Job drawing, mm, ordinate dimensions from the low corner. One solid piece. A direction names the side the tool comes from. Give positions to 0.01 mm unless a question says otherwise; leave off trailing zeros. Write each loop counter-clockwise with the first axis right and the second up, starting at its lowest first coordinate (ties: lowest second). Pieces come first, ordered by that corner, then holes. Notation, with made-up numbers: (79.5, 16.5) - (107.5, 16.5) arc R7 cw to (107.5, 24.5) - close; hole circle Ø5 at (-28.75, 55). An arc over 180 degrees is marked (long way). Use a Markdown table: item, result. Add a question column.
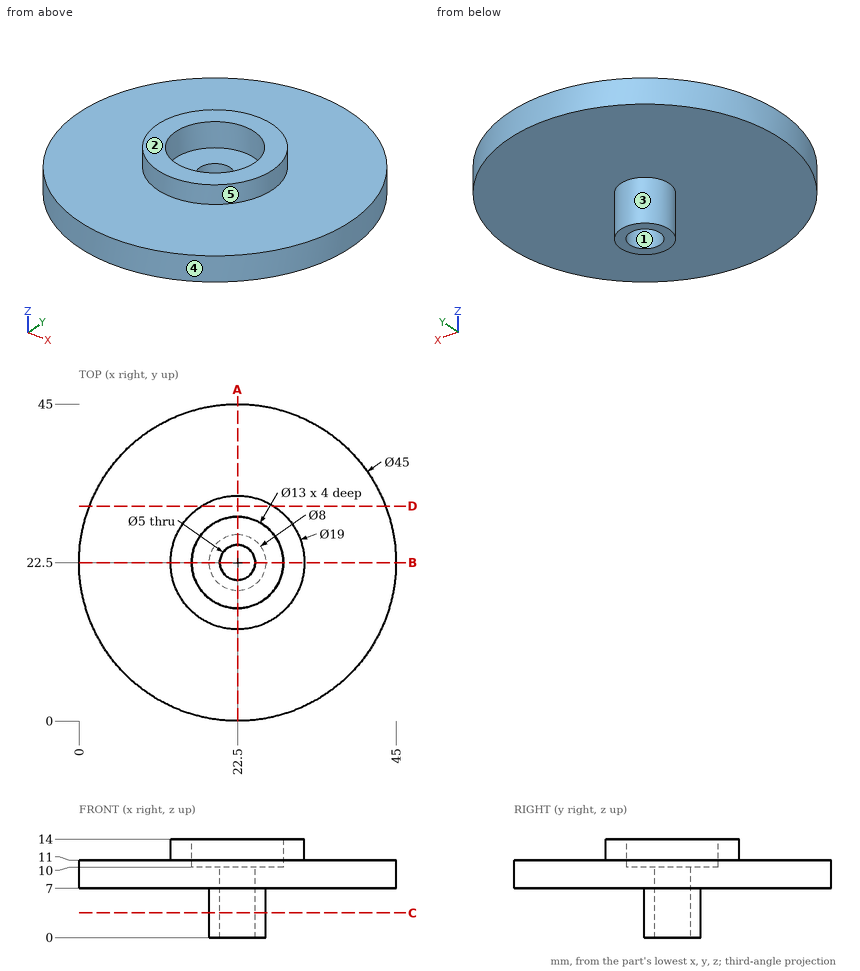
(1) Band-saw the part on C-C (z = 3.5). Write the cut outline in (x, y), then the cut area to 3 significant figures.
(2) Flat gauge pins, fed straight in: pin 1 (1 mm diameter, centred on y = 35.5, z = 9, fed in from -X); pin 2 (6 mm diameter, centred on y = 26, z = 7, fed in from -X); pin 3 (6 mm diameter, centred on y = 7.5, z = 12, fed in from +X). Where does each tip first touch, or does it go through?
(3) Band-saw the part on D-D (y = 30.5). Write the cut outline in (x, z).
(4) Probe probe 1 along X at (y, z) = (22.5, 12.9); probe 2 along Z at (x, y) = (30.5, 30); probe 3 along X at (y, z) = (22.5, 4.5). List the from-to ranges inside material, lowest first. Write a range as [from, to].
(5) Two-plate mould, pull along X, no slides. Class the marked faces 1, 2 and 3: +X half, -X half, draft (parallel to the pull), parting line (faces both ways), or undercut.
(6) Which spindle directions (+Z, -Z, +X, -X, +Y, -Y) get a long thin tool onto all of the face, cutting with end or side? Do the marked faces 4 and 5. Say none if no direction does.
(7) Band-saw the part on A-A (x = 22.5). Write the cut outline in (y, z).
Model answer:
| question | item | result |
|---|---|---|
| 1 | outline | circle Ø8 at (22.5, 22.5); hole circle Ø5 at (22.5, 22.5) |
| 1 | area | 30.6 mm^2 |
| 2 | pin 1 | stops at x = 3.79 |
| 2 | pin 2 | stops at x = 0.01 |
| 2 | pin 3 | stops at x = 41.42 |
| 3 | outline | (1.47, 7) - (43.53, 7) - (43.53, 11) - (27.62, 11) - (27.62, 14) - (17.38, 14) - (17.38, 11) - (1.47, 11) - close |
| 4 | probe 1 | x = [13, 16], [29, 32] |
| 4 | probe 2 | z = [7, 11] |
| 4 | probe 3 | x = [18.5, 20], [25, 26.5] |
| 5 | face 1 | undercut |
| 5 | face 2 | draft |
| 5 | face 3 | parting line |
| 6 | face 4 | +Z, -Z |
| 6 | face 5 | +Z |
| 7 | outline | (0, 7) - (18.5, 7) - (18.5, 0) - (20, 0) - (20, 10) - (16, 10) - (16, 14) - (13, 14) - (13, 11) - (0, 11) - close; (25, 0) - (26.5, 0) - (26.5, 7) - (45, 7) - (45, 11) - (32, 11) - (32, 14) - (29, 14) - (29, 10) - (25, 10) - close |
